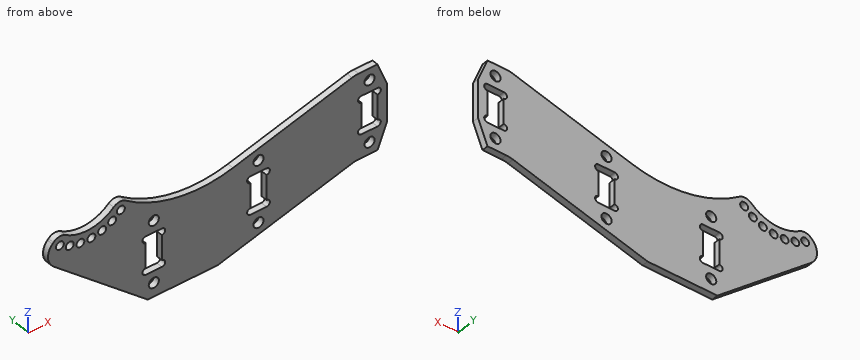
Autodesk Inventor part; units mm, degrees
ref_plane "YZ Plane" through (0, 0, 0) normal (1, 0, 0) x (0, 1, 0)
ref_plane "XZ Plane" through (0, 0, 0) normal (0, 1, 0) x (-1, 0, 0)
ref_plane "XY Plane" through (0, 0, 0) normal (0, 0, 1) x (1, 0, 0)
sketch "スケッチ1" plane through (0, 0, 0) normal (0, 1, 0) x (-1, 0, 0)
  line L0 (0, 0) -> (7, 0)
  line L1 (7, 0) -> (7, -27) construction
  line L2 (7, -27) -> (0, -27)
  line L3 (0, -27) -> (0, 0) construction
  circle A0 centre (2.5, -3.7) radius 1.6
  circle A1 centre (2.5, -23.3) radius 1.6
  line L4 (5.05, -7.5) -> (0.05, -7.5) construction
  line L5 (0.05, -7.5) -> (0.05, -19.5) construction
  line L6 (0.05, -19.5) -> (5.05, -19.5) construction
  line L7 (5.05, -19.5) -> (5.05, -7.5) construction
  line L8 (0, -7.45) -> (5.1, -7.45)
  line L9 (5.1, -7.45) -> (5.1, -19.55)
  line L10 (5.1, -19.55) -> (0, -19.55)
  line L11 (0, -19.55) -> (0, -7.45)
  line L12 (84.5459, 21.5815) -> (61.9185, -1.0459) construction
  line L13 (61.9185, -1.0459) -> (65.4541, -4.5815) construction
  line L14 (65.4541, -4.5815) -> (88.0815, 18.0459) construction
  line L15 (88.0815, 18.0459) -> (84.5459, 21.5815) construction
  line L16 (70.3953, 0.3598) -> (83.1317, 13.0962)
  circle A2 centre (100.1023, -8.117) radius 1.25
  line L17 (7, 0) -> (45.561, -10.3324)
  line L18 (7, -27) -> (50.4418, -38.6402)
  line L19 (72.4418, -38.6402) -> (106.1477, -10.3575)
  line L20 (106.1477, -10.3575) -> (100.2529, -4.1751)
  arc A3 (45.561, -10.3324) -> (81.4937, -2.447) centre (55.9138, 28.3046) ccw
  line L21 (72.4418, -38.6402) -> (50.4418, -38.6402)
  line L22 (40, -9.2) -> (35, -9.2) construction
  line L23 (35, -9.2) -> (35, -34.2) construction
  line L24 (35, -34.2) -> (40, -34.2) construction
  line L25 (40, -34.2) -> (40, -9.2) construction
  circle A4 centre (97.0056, -9.675) radius 1.25
  circle A5 centre (93.6401, -10.5063) radius 1.25
  circle A6 centre (90.1742, -10.5693) radius 1.25
  circle A7 centre (86.7807, -9.8609) radius 1.25
  circle A8 centre (83.6295, -8.4164) radius 1.25
  circle A9 centre (80.8777, -6.3081) radius 1.25
  line L26 (100.2529, -4.1751) -> (104.1748, -8.2883)
  arc A10 (81.4937, -2.447) -> (100.2529, -4.1751) centre (91.6271, 4.8718) ccw
  line L27 (40, -15.7) -> (35, -15.7) construction
  line L28 (35, -15.7) -> (35, -27.7) construction
  line L29 (35, -27.7) -> (40, -27.7) construction
  line L30 (40, -27.7) -> (40, -15.7) construction
  line L31 (34.95, -15.65) -> (40.05, -15.65)
  line L32 (40.05, -15.65) -> (40.05, -27.75)
  line L33 (40.05, -27.75) -> (34.95, -27.75)
  line L34 (34.95, -27.75) -> (34.95, -15.65)
  circle A11 centre (37.5, -11.9) radius 1.6
  circle A12 centre (37.5, -31.5) radius 1.6
  line L35 (73, -12) -> (68, -12) construction
  line L36 (68, -12) -> (68, -37) construction
  line L37 (68, -37) -> (73, -37) construction
  line L38 (73, -37) -> (73, -12) construction
  line L39 (73, -18.5) -> (68, -18.5) construction
  line L40 (68, -18.5) -> (68, -30.5) construction
  line L41 (68, -30.5) -> (73, -30.5) construction
  line L42 (73, -30.5) -> (73, -18.5) construction
  line L43 (67.95, -18.45) -> (73.05, -18.45)
  line L44 (73.05, -18.45) -> (73.05, -30.55)
  line L45 (73.05, -30.55) -> (67.95, -30.55)
  line L46 (67.95, -30.55) -> (67.95, -18.45)
  circle A13 centre (70.5, -14.7) radius 1.6
  circle A14 centre (70.5, -34.3) radius 1.6
  circle A15 centre (73.05, -19.5) radius 1.05
  circle A16 centre (67.95, -19.5) radius 1.05
  circle A17 centre (67.95, -29.5) radius 1.05
  circle A18 centre (73.05, -29.5) radius 1.05
  circle A19 centre (40.05, -16.7) radius 1.05
  circle A20 centre (34.95, -16.7) radius 1.05
  circle A21 centre (34.95, -26.7) radius 1.05
  circle A22 centre (40.05, -26.7) radius 1.05
  circle A23 centre (5.1, -8.5) radius 1.05
  circle A24 centre (0, -8.5) radius 1.05
  circle A25 centre (0, -18.5) radius 1.05
  circle A26 centre (5.1, -18.5) radius 1.05
  line L47 (-3, -7.45) -> (-3, -19.55)
  line L48 (-3, -19.55) -> (0, -27)
  line L49 (-3, -7.45) -> (0, 0)
  circle A27 centre (91.6271, 4.8718) radius 15.5
  point P0 (75, 8.5)
  point P1 (91.6085, -20.8534)
  point P2 (82.042, -3.1517)
  point P3 (81.2596, -2.6403)
  point P4 (55.561, -0.3324)
  point P5 (40, -14.6)
  point P6 (35, -14.6)
  point P7 (40, -28.8)
  point P8 (35, -28.8)
  dimension "d0" = 7
  dimension "d1" = 27
  dimension "d2" = 3.2
  dimension "d3" = 3.2
  dimension "d4" = 5
  dimension "d5" = 12
  dimension "d6" = 2.5
  dimension "d7" = 2.5
  dimension "d8" = 19.6
  dimension "d9" = 3.7
  dimension "d11" = 7.5
  dimension "d12" = 0.05
  dimension "d20" = 32
  dimension "d21" = 5
  dimension "d22" = 45
  dimension "d23" = 2.5
  dimension "d24" = 16
  dimension "d25" = 75
  dimension "d26" = 8.5
  dimension "d27" = 30
  dimension "d33" = 27
  dimension "d35" = 2.5
  dimension "d44" = 75
  dimension "d49" = 75
  dimension "d52" = 40
  dimension "d53" = 30
  dimension "d56" = 39
  dimension "d61" = 5
  dimension "d62" = 25
  dimension "d63" = 33
  dimension "d64" = 9.2
  dimension "d69" = 77
  dimension "d72" = 22
  dimension "d73" = 12.5
  dimension "d74" = 50
  dimension "d75" = 21
  dimension "d76" = 44
  dimension "d77" = 12
  dimension "d78" = 6.5
  dimension "d79" = 0.05
  dimension "d84" = 3.2
  dimension "d85" = 2.5
  dimension "d86" = 2.7
  dimension "d88" = 3.2
  dimension "d89" = 19.6
  dimension "d90" = 2.5
  dimension "d91" = 5
  dimension "d92" = 25
  dimension "d93" = 12
  dimension "d94" = 6.5
  dimension "d95" = 0.05
  dimension "d100" = 3.2
  dimension "d101" = 2.5
  dimension "d102" = 2.7
  dimension "d104" = 3.2
  dimension "d105" = 19.6
  dimension "d106" = 2.5
  dimension "d107" = 12
  dimension "d109" = 66
  dimension "d118" = 2.1
  dimension "d119" = 2.1
  dimension "d120" = 2.1
  dimension "d121" = 2.1
  dimension "d122" = 2.1
extrude "押し出し2" add sketch "スケッチ1" along normal blind 2 contours L0 L17 A3 A27 A9 A8 A7 A6 A5 A4 A2 L20 L19 L21 L18 L2 L48 L47 L49 | A3 A10 L20 A27 A2 A4 A5 A6 A7 A8 A9
fillet "フィレット1" radius 5 1 edges at (-106.1477, 1, -10.3575)
fillet "フィレット2" radius 3 2 edges at (-81.4937, 1, -2.447) (-100.2529, 1, -4.1751)
fillet "フィレット3" radius 8 2 edges at (-7, 1, -27) (-7, 1, 0)
equation "\"d7\" = d6"
equation "\"d11\" = -0.5 * d5 + 0.5 * d1"
equation "\"d49\" = d44"
equation "\"d28\" = d20 - 2 * d29"
properties part number "頭＿メインフレーム" material "GFRP"
Design review of the part built by this model. Coordinates are the model's own, in mm. Give positions to 0.01 mm unless a question says otherwise; leave off trailing zeros. Write each loop counter-clockwise with the first axis right and the second up, starting at its lowest first coordinate (ties: lowest second). Pieces come first, ordered by that corner, then holes.
(1) Add section B-B (x = -37.5). Give the boundary of the cut face in (y, z), and give its area (3 significant figures).
Checked values:
outline: (0, -35.17) - (2, -35.17) - (2, -33.1) - (0, -33.1) - close; (0, -29.9) - (2, -29.9) - (2, -27.75) - (0, -27.75) - close; (0, -15.65) - (2, -15.65) - (2, -13.5) - (0, -13.5) - close; (0, -10.3) - (2, -10.3) - (2, -8.17) - (0, -8.17) - close
area: 17.0 mm2
(2) Add section A-A (z = -31.5). Give the boundary of the cut face in (x, y), and give its area (3 significant figures).
Checked values:
outline: (-80.95, 0) - (-39.1, 0) - (-39.1, 2) - (-80.95, 2) - close; (-35.9, 0) - (-23.79, 0) - (-23.79, 2) - (-35.9, 2) - close
area: 108 mm2
(3) Wall thickness on line 1 along Z through (x, y) = (-71, 0.8); line 2 along X through (y, z) = (1.3, -13); line 3 along X through (y, z) = (0.55, -24.5): over which ranges is each line inside the solid? List them lowest first.
Checked values:
line 1: z = -38.64 to -35.82, -32.78 to -30.55, -18.45 to -16.22, -13.18 to -8.74
line 2: x = -102.82 to -38.66, -36.34 to -5.1, 0 to 3
line 3: x = -89.29 to -73.05, -67.95 to -40.05, -34.95 to -3.56, -1.44 to 1.01
(4) Clearance check with flat-ended pins moving along their axes: pin 1 Ø2.5 at (x, z) = (-2.5, -23.3) entering from -Y; pin 2 Ø1 at (y, z) = (1, -20.5) entering from -X. State where each tip first meets the part, or that it passes through.
Checked values:
pin 1: passes through
pin 2: stops at x = -94.66
(5) Add section D-D (y = 0.85). Give the number of separate pieces and of enclosed holes in the cut face, and give its area (3 significant figures).
Checked values:
separate pieces: 1
enclosed holes: 16
area: 2,350 mm2
(6) Add section C-C (x = -76.5). Give the boundary of the cut face in (y, z).
Checked values:
outline: (0, -35.23) - (2, -35.23) - (2, -5.99) - (0, -5.99) - close
